from build123d import *

# Parameters (mm, degrees)
ESQUISSE1_W                     = 355.6
ESQUISSE1_H                     = 107.95
BOSS_EXTRU_1_DEPTH              = 6.35
ESQUISSE4_W                     = 6.35
ESQUISSE4_H                     = 10.16
ENL_V_MAT_EXTRU_3_DEPTH         = 6.35
R_P_TITION_LIN_AIRE2_COUNT      = 7
R_P_TITION_LIN_AIRE2_PITCH      = 20.32
R_P_TITION_LIN_AIRE2_COUNT_DIR2 = 2
R_P_TITION_LIN_AIRE2_PITCH_DIR2 = 349.25
ESQUISSE5_W                     = 25.4
ESQUISSE5_H                     = 6.35
ENL_V_MAT_EXTRU_4_DEPTH         = 6.35
R_P_TITION_LIN_AIRE3_COUNT      = 7
R_P_TITION_LIN_AIRE3_PITCH      = 50.8
ESQUISSE6_W                     = 12.7
ESQUISSE6_H                     = 6.35
ENL_V_MAT_EXTRU_5_DEPTH         = 6.35
ESQUISSE8_W                     = 12.7
ESQUISSE8_H                     = 6.35
ENL_V_MAT_EXTRU_7_DEPTH         = 6.35
ESQUISSE9_W                     = 25.4
ESQUISSE9_H                     = 6.35
ENL_V_MAT_EXTRU_8_DEPTH         = 6.35
R_P_TITION_LIN_AIRE6_COUNT      = 7
R_P_TITION_LIN_AIRE6_PITCH      = 50.8


with BuildPart() as part:
    # Esquisse1 → Boss.-Extru.1 (new body)
    with BuildSketch(Plane.XY):
        Rectangle(ESQUISSE1_W, ESQUISSE1_H)
    extrude(amount=BOSS_EXTRU_1_DEPTH)

    # Esquisse4 → Enlèv. mat.-Extru.3 (cut)
    with BuildSketch(Plane.XY.offset(6.35)):
        with Locations((-174.625, 38.735)):
            Rectangle(ESQUISSE4_W, ESQUISSE4_H)
    enl_v_mat_extru_3 = extrude(amount=-ENL_V_MAT_EXTRU_3_DEPTH, mode=Mode.SUBTRACT)

    # Répétition linéaire2: Enl_v. mat.-Extru.3 7 × 2
    with Locations(*[(j * R_P_TITION_LIN_AIRE2_PITCH_DIR2, -i * R_P_TITION_LIN_AIRE2_PITCH, 0) for i in range(R_P_TITION_LIN_AIRE2_COUNT) for j in range(R_P_TITION_LIN_AIRE2_COUNT_DIR2) if (i, j) != (0, 0)]):
        add(enl_v_mat_extru_3, mode=Mode.SUBTRACT)

    # Esquisse5 → Enlèv. mat.-Extru.4 (cut)
    with BuildSketch(Plane.XY.offset(6.35)):
        with Locations((-152.4, -50.8)):
            Rectangle(ESQUISSE5_W, ESQUISSE5_H)
    enl_v_mat_extru_4 = extrude(amount=-ENL_V_MAT_EXTRU_4_DEPTH, mode=Mode.SUBTRACT)

    # Répétition linéaire3: Enlèv. mat.-Extru.4 ×7
    with Locations(*[(i * R_P_TITION_LIN_AIRE3_PITCH, 0, 0) for i in range(1, R_P_TITION_LIN_AIRE3_COUNT)]):
        add(enl_v_mat_extru_4, mode=Mode.SUBTRACT)

    # Esquisse6 → Enlèv. mat.-Extru.5 (cut)
    with BuildSketch(Plane.XY.offset(6.35)):
        with Locations((-171.45, -50.8)):
            Rectangle(ESQUISSE6_W, ESQUISSE6_H)
    extrude(amount=-ENL_V_MAT_EXTRU_5_DEPTH, mode=Mode.SUBTRACT)

    # Esquisse8 → Enlèv. mat.-Extru.7 (cut)
    with BuildSketch(Plane.XY.offset(6.35)):
        with Locations((171.45, -50.8)):
            Rectangle(ESQUISSE8_W, ESQUISSE8_H)
    extrude(amount=-ENL_V_MAT_EXTRU_7_DEPTH, mode=Mode.SUBTRACT)

    # Esquisse9 → Enlèv. mat.-Extru.8 (cut)
    with BuildSketch(Plane.XY.offset(6.35)):
        with Locations((-152.4, 0)):
            Rectangle(ESQUISSE9_W, ESQUISSE9_H)
    enl_v_mat_extru_8 = extrude(amount=-ENL_V_MAT_EXTRU_8_DEPTH, mode=Mode.SUBTRACT)

    # Répétition linéaire6: Enlèv. mat.-Extru.8 ×7
    with Locations(*[(i * R_P_TITION_LIN_AIRE6_PITCH, 0, 0) for i in range(1, R_P_TITION_LIN_AIRE6_COUNT)]):
        add(enl_v_mat_extru_8, mode=Mode.SUBTRACT)


solid = part.part
Input: part model. Units: mm. Frame: model coordinates. A direction names the side the tool comes from. Give positions to 0.01 mm unless a question says otherwise; leave off trailing zeros. Write each loop counter-clockwise with the first axis right and the second up, starting at its lowest first coordinate (ties: lowest second). Pieces come first, ordered by that corner, then holes.
Q1. Material intervals for probe 1 along X at (y, z) = (21, 4.75); probe 2 along Y at (x, z) = (-9.5, 1.25) (3 decimals), sorted ascending.
Q2. First-contact query: P1, Ø1.5, axis at x = 92, z = 4, coming from the -Y side (3 decimals); P2, Ø1, axis at y = 15.5, z = 2, coming from the +X side; P3, Ø1.9, axis at y = 1.5, z = 2.5, coming from the -X side. Flat tips, straight axial feed; report the tip coordinate or a pass-through.
Q3. Section B-B, the plane z = 2.75. State how many separate pieces and enclosed holes the cut face has, plus the area to 3 significant figures.
Q4. Set-up query: faces 4 (the face through (-102, -3.175, 3)), 5 (the face through (-175, 13.335, 3)), 6 (the face through (175, -27.305, 3)). Return all of +Z, -Z, +X, -X, +Y, -Y with unobstructed straight access to the full face (end or side cutting, diameter ignored); none if empty.
Q5. Section A-A, the plane x = -155. Output: boundary loops of the cut face in (y, z) (3 decimals), plus the area to 3 significant figures.
Q6. Section C-C, the plane y = -22. Output: boundary loops of the cut face in (x, z), plus the area to 3 significant figures.
Q7. Pull-direction query (X, two-part tool) for faces 1 (the face through (-177.8, 8, 3)), 2 (the face through (-2, 13, 6.35)), 3 (the face through (114.3, 0, 3)); classes: pulls with the +X half, pulls with the -X half, needs draft (parallel to the pull), parting line crosses it, or undercut.
Filled in:
1. probe 1: x = -171.45 to 171.45
1. probe 2: y = -47.625 to -3.175, 3.175 to 53.975
2. P1: stops at y = -47.625
2. P2: stops at x = 171.45
2. P3: stops at x = -171.45
3. separate pieces: 1
3. enclosed holes: 7
3. area: 35,300 mm2
4. face 4: +Z, -Z
4. face 5: +Z, -Z, -X
4. face 6: +Z, -Z, +X
5. outline: (-47.625, 0) - (-3.175, 0) - (-3.175, 6.35) - (-47.625, 6.35) - close; (3.175, 0) - (53.975, 0) - (53.975, 6.35) - (3.175, 6.35) - close
5. area: 605 mm2
6. outline: (-171.45, 0) - (171.45, 0) - (171.45, 6.35) - (-171.45, 6.35) - close
6. area: 2,180 mm2
7. face 1: pulls with the -X half
7. face 2: needs draft
7. face 3: undercut
